The listing builds one solid part. Answer for the finished solid, in the listing's coordinates (mm). A direction names the side the tool comes from. Coordinates: 2 decimals unless noted, no trailing zeros. Write each loop counter-clockwise with the first axis right and the second up, starting at its lowest first coordinate (ties: lowest second). Pieces come first, ordered by that corner, then holes.
from build123d import *

# Parameters (mm, degrees)
SKETCH1_R           = 25.4
SKETCH1_R_2         = 3.175
BOSS_EXTRUDE1_DEPTH = 2.54
SKETCH2_R           = 3.175
BOSS_EXTRUDE4_DEPTH = 13.97
SKETCH5_R           = 3.175
BOSS_EXTRUDE6_DEPTH = 2.54
SKETCH5_4_R         = 11.1125
BOSS_EXTRUDE7_DEPTH = 8.89
SKETCH6_R           = 25.4
SKETCH6_R_2         = 11.1125
BOSS_EXTRUDE8_DEPTH = 2.54


with BuildPart() as part:
    # Sketch1 → Boss-Extrude1 (new body)
    with BuildSketch(Plane(origin=(0, 0, 0), x_dir=(1, 0, 0), z_dir=(0, 1, 0))):
        Circle(SKETCH1_R)
        Circle(SKETCH1_R_2, mode=Mode.SUBTRACT)
    extrude(amount=BOSS_EXTRUDE1_DEPTH)

    # Sketch2 → Boss-Extrude4 (add)
    with BuildSketch(Plane(origin=(0, 2.54, 0), x_dir=(1, 0, 0), z_dir=(0, 1, 0))):
        with BuildLine():
            ThreePointArc((0.635, 25.392061259), (0, 25.4), (-0.635, 25.392061259))
            Line((-0.635, 25.392061259), (-0.635, 4.719976827))
            ThreePointArc((-0.635, 4.719976827), (-1.822529847, 4.399976274), (-2.888514816, 3.786540428))
            Line((-2.888514816, 3.786540428), (-17.505885899, 18.403911511))
            ThreePointArc((-17.505885899, 18.403911511), (-17.960512242, 17.960512242), (-18.403911511, 17.505885899))
            Line((-18.403911511, 17.505885899), (-3.786540428, 2.888514816))
            ThreePointArc((-3.786540428, 2.888514816), (-4.399976274, 1.822529847), (-4.719976827, 0.635))
            Line((-4.719976827, 0.635), (-25.392061259, 0.635))
            ThreePointArc((-25.392061259, 0.635), (-25.4, 0), (-25.392061259, -0.635))
            Line((-25.392061259, -0.635), (-4.719976827, -0.635))
            ThreePointArc((-4.719976827, -0.635), (-4.399976274, -1.822529847), (-3.786540428, -2.888514816))
            Line((-3.786540428, -2.888514816), (-18.403911511, -17.505885899))
            ThreePointArc((-18.403911511, -17.505885899), (-17.960512242, -17.960512242), (-17.505885899, -18.403911511))
            Line((-17.505885899, -18.403911511), (-2.888514816, -3.786540428))
            ThreePointArc((-2.888514816, -3.786540428), (-1.822529847, -4.399976274), (-0.635, -4.719976827))
            Line((-0.635, -4.719976827), (-0.635, -25.392061259))
            ThreePointArc((-0.635, -25.392061259), (0, -25.4), (0.635, -25.392061259))
            Line((0.635, -25.392061259), (0.635, -4.719976827))
            ThreePointArc((0.635, -4.719976827), (1.822529847, -4.399976274), (2.888514816, -3.786540428))
            Line((2.888514816, -3.786540428), (17.505885899, -18.403911511))
            ThreePointArc((17.505885899, -18.403911511), (17.960512242, -17.960512242), (18.403911511, -17.505885899))
            Line((18.403911511, -17.505885899), (3.786540428, -2.888514816))
            ThreePointArc((3.786540428, -2.888514816), (4.399976274, -1.822529847), (4.719976827, -0.635))
            Line((4.719976827, -0.635), (25.392061259, -0.635))
            ThreePointArc((25.392061259, -0.635), (25.4, 0), (25.392061259, 0.635))
            Line((25.392061259, 0.635), (4.719976827, 0.635))
            ThreePointArc((4.719976827, 0.635), (4.399976274, 1.822529847), (3.786540428, 2.888514816))
            Line((3.786540428, 2.888514816), (18.403911511, 17.505885899))
            ThreePointArc((18.403911511, 17.505885899), (17.960512242, 17.960512242), (17.505885899, 18.403911511))
            Line((17.505885899, 18.403911511), (2.888514816, 3.786540428))
            ThreePointArc((2.888514816, 3.786540428), (1.822529847, 4.399976274), (0.635, 4.719976827))
            Line((0.635, 4.719976827), (0.635, 25.392061259))
        make_face()
        Circle(SKETCH2_R, mode=Mode.SUBTRACT)
    extrude(amount=BOSS_EXTRUDE4_DEPTH)

    # Sketch5 → Boss-Extrude6 (add)
    with BuildSketch(Plane(origin=(0, 16.51, 0), x_dir=(1, 0, 0), z_dir=(0, 1, 0))):
        with BuildLine():
            Line((3.786540428, -2.888514816), (8.293897485, -7.395871873))
            ThreePointArc((8.293897485, -7.395871873), (10.266611305, -4.252569642), (11.094342308, -0.635))
            Line((11.094342308, -0.635), (4.719976827, -0.635))
            ThreePointArc((4.719976827, -0.635), (4.399976274, -1.822529847), (3.786540428, -2.888514816))
        make_face()
        with BuildLine():
            ThreePointArc((-0.635, -11.094342308), (0, -11.1125), (0.635, -11.094342308))
            Line((0.635, -11.094342308), (0.635, -4.719976827))
            ThreePointArc((0.635, -4.719976827), (1.822529847, -4.399976274), (2.888514816, -3.786540428))
            Line((2.888514816, -3.786540428), (7.395871873, -8.293897485))
            ThreePointArc((7.395871873, -8.293897485), (7.857724106, -7.857724106), (8.293897485, -7.395871873))
            Line((8.293897485, -7.395871873), (3.786540428, -2.888514816))
            ThreePointArc((3.786540428, -2.888514816), (4.399976274, -1.822529847), (4.719976827, -0.635))
            Line((4.719976827, -0.635), (11.094342308, -0.635))
            ThreePointArc((11.094342308, -0.635), (11.107959649, -0.317629777), (11.1125, 0))
            ThreePointArc((11.1125, 0), (11.107959649, 0.317629777), (11.094342308, 0.635))
            Line((11.094342308, 0.635), (4.719976827, 0.635))
            ThreePointArc((4.719976827, 0.635), (4.399976274, 1.822529847), (3.786540428, 2.888514816))
            Line((3.786540428, 2.888514816), (8.293897485, 7.395871873))
            ThreePointArc((8.293897485, 7.395871873), (7.857724106, 7.857724106), (7.395871873, 8.293897485))
            Line((7.395871873, 8.293897485), (2.888514816, 3.786540428))
            ThreePointArc((2.888514816, 3.786540428), (1.822529847, 4.399976274), (0.635, 4.719976827))
            Line((0.635, 4.719976827), (0.635, 11.094342308))
            ThreePointArc((0.635, 11.094342308), (0, 11.1125), (-0.635, 11.094342308))
            Line((-0.635, 11.094342308), (-0.635, 4.719976827))
            ThreePointArc((-0.635, 4.719976827), (-1.822529847, 4.399976274), (-2.888514816, 3.786540428))
            Line((-2.888514816, 3.786540428), (-7.395871873, 8.293897485))
            ThreePointArc((-7.395871873, 8.293897485), (-7.857724106, 7.857724106), (-8.293897485, 7.395871873))
            Line((-8.293897485, 7.395871873), (-3.786540428, 2.888514816))
            ThreePointArc((-3.786540428, 2.888514816), (-4.399976274, 1.822529847), (-4.719976827, 0.635))
            Line((-4.719976827, 0.635), (-11.094342308, 0.635))
            ThreePointArc((-11.094342308, 0.635), (-11.1125, 0), (-11.094342308, -0.635))
            Line((-11.094342308, -0.635), (-4.719976827, -0.635))
            ThreePointArc((-4.719976827, -0.635), (-4.399976274, -1.822529847), (-3.786540428, -2.888514816))
            Line((-3.786540428, -2.888514816), (-8.293897485, -7.395871873))
            ThreePointArc((-8.293897485, -7.395871873), (-7.857724106, -7.857724106), (-7.395871873, -8.293897485))
            Line((-7.395871873, -8.293897485), (-2.888514816, -3.786540428))
            ThreePointArc((-2.888514816, -3.786540428), (-1.822529847, -4.399976274), (-0.635, -4.719976827))
            Line((-0.635, -4.719976827), (-0.635, -11.094342308))
        make_face()
        Circle(SKETCH5_R, mode=Mode.SUBTRACT)
        with BuildLine():
            Line((0.635, -4.719976827), (0.635, -11.094342308))
            ThreePointArc((0.635, -11.094342308), (4.252569642, -10.266611305), (7.395871873, -8.293897485))
            Line((7.395871873, -8.293897485), (2.888514816, -3.786540428))
            ThreePointArc((2.888514816, -3.786540428), (1.822529847, -4.399976274), (0.635, -4.719976827))
        make_face()
        with BuildLine():
            ThreePointArc((-7.395871873, -8.293897485), (-4.252569642, -10.266611305), (-0.635, -11.094342308))
            Line((-0.635, -11.094342308), (-0.635, -4.719976827))
            ThreePointArc((-0.635, -4.719976827), (-1.822529847, -4.399976274), (-2.888514816, -3.786540428))
            Line((-2.888514816, -3.786540428), (-7.395871873, -8.293897485))
        make_face()
        with BuildLine():
            ThreePointArc((-11.094342308, -0.635), (-10.266611305, -4.252569642), (-8.293897485, -7.395871873))
            Line((-8.293897485, -7.395871873), (-3.786540428, -2.888514816))
            ThreePointArc((-3.786540428, -2.888514816), (-4.399976274, -1.822529847), (-4.719976827, -0.635))
            Line((-4.719976827, -0.635), (-11.094342308, -0.635))
        make_face()
        with BuildLine():
            ThreePointArc((-8.293897485, 7.395871873), (-10.266611305, 4.252569642), (-11.094342308, 0.635))
            Line((-11.094342308, 0.635), (-4.719976827, 0.635))
            ThreePointArc((-4.719976827, 0.635), (-4.399976274, 1.822529847), (-3.786540428, 2.888514816))
            Line((-3.786540428, 2.888514816), (-8.293897485, 7.395871873))
        make_face()
        with BuildLine():
            ThreePointArc((-0.635, 11.094342308), (-4.252569642, 10.266611305), (-7.395871873, 8.293897485))
            Line((-7.395871873, 8.293897485), (-2.888514816, 3.786540428))
            ThreePointArc((-2.888514816, 3.786540428), (-1.822529847, 4.399976274), (-0.635, 4.719976827))
            Line((-0.635, 4.719976827), (-0.635, 11.094342308))
        make_face()
        with BuildLine():
            Line((2.888514816, 3.786540428), (7.395871873, 8.293897485))
            ThreePointArc((7.395871873, 8.293897485), (4.252569642, 10.266611305), (0.635, 11.094342308))
            Line((0.635, 11.094342308), (0.635, 4.719976827))
            ThreePointArc((0.635, 4.719976827), (1.822529847, 4.399976274), (2.888514816, 3.786540428))
        make_face()
        with BuildLine():
            Line((4.719976827, 0.635), (11.094342308, 0.635))
            ThreePointArc((11.094342308, 0.635), (10.266611305, 4.252569642), (8.293897485, 7.395871873))
            Line((8.293897485, 7.395871873), (3.786540428, 2.888514816))
            ThreePointArc((3.786540428, 2.888514816), (4.399976274, 1.822529847), (4.719976827, 0.635))
        make_face()
    extrude(amount=BOSS_EXTRUDE6_DEPTH)

    # Sketch5_4 → Boss-Extrude7 (add)
    with BuildSketch(Plane(origin=(0, 16.51, 0), x_dir=(1, 0, 0), z_dir=(0, 1, 0))):
        with BuildLine():
            Line((-0.635, -12.684115066), (-0.635, -25.392061259))
            ThreePointArc((-0.635, -25.392061259), (0, -25.4), (0.635, -25.392061259))
            Line((0.635, -25.392061259), (0.635, -12.684115066))
            ThreePointArc((0.635, -12.684115066), (4.860079591, -11.733270063), (8.52001097, -9.418036582))
            Line((8.52001097, -9.418036582), (17.505885899, -18.403911511))
            ThreePointArc((17.505885899, -18.403911511), (17.960512242, -17.960512242), (18.403911511, -17.505885899))
            Line((18.403911511, -17.505885899), (9.418036582, -8.52001097))
            ThreePointArc((9.418036582, -8.52001097), (11.733270063, -4.860079591), (12.684115066, -0.635))
            Line((12.684115066, -0.635), (25.392061259, -0.635))
            ThreePointArc((25.392061259, -0.635), (25.4, 0), (25.392061259, 0.635))
            Line((25.392061259, 0.635), (12.684115066, 0.635))
            ThreePointArc((12.684115066, 0.635), (11.733270063, 4.860079591), (9.418036582, 8.52001097))
            Line((9.418036582, 8.52001097), (18.403911511, 17.505885899))
            ThreePointArc((18.403911511, 17.505885899), (17.960512242, 17.960512242), (17.505885899, 18.403911511))
            Line((17.505885899, 18.403911511), (8.52001097, 9.418036582))
            ThreePointArc((8.52001097, 9.418036582), (4.860079591, 11.733270063), (0.635, 12.684115066))
            Line((0.635, 12.684115066), (0.635, 25.392061259))
            ThreePointArc((0.635, 25.392061259), (0, 25.4), (-0.635, 25.392061259))
            Line((-0.635, 25.392061259), (-0.635, 12.684115066))
            ThreePointArc((-0.635, 12.684115066), (-4.860079591, 11.733270063), (-8.52001097, 9.418036582))
            Line((-8.52001097, 9.418036582), (-17.505885899, 18.403911511))
            ThreePointArc((-17.505885899, 18.403911511), (-17.960512242, 17.960512242), (-18.403911511, 17.505885899))
            Line((-18.403911511, 17.505885899), (-9.418036582, 8.52001097))
            ThreePointArc((-9.418036582, 8.52001097), (-11.733270063, 4.860079591), (-12.684115066, 0.635))
            Line((-12.684115066, 0.635), (-25.392061259, 0.635))
            ThreePointArc((-25.392061259, 0.635), (-25.4, 0), (-25.392061259, -0.635))
            Line((-25.392061259, -0.635), (-12.684115066, -0.635))
            ThreePointArc((-12.684115066, -0.635), (-11.733270063, -4.860079591), (-9.418036582, -8.52001097))
            Line((-9.418036582, -8.52001097), (-18.403911511, -17.505885899))
            ThreePointArc((-18.403911511, -17.505885899), (-17.960512242, -17.960512242), (-17.505885899, -18.403911511))
            Line((-17.505885899, -18.403911511), (-8.52001097, -9.418036582))
            ThreePointArc((-8.52001097, -9.418036582), (-4.860079591, -11.733270063), (-0.635, -12.684115066))
        make_face()
        Circle(SKETCH5_4_R, mode=Mode.SUBTRACT)
    extrude(amount=BOSS_EXTRUDE7_DEPTH)

    # Sketch6 → Boss-Extrude8 (add)
    with BuildSketch(Plane(origin=(0, 25.4, 0), x_dir=(1, 0, 0), z_dir=(0, 1, 0))):
        Circle(SKETCH6_R)
        Circle(SKETCH6_R_2, mode=Mode.SUBTRACT)
    extrude(amount=BOSS_EXTRUDE8_DEPTH)


solid = part.part
Q1. Find the intervals of material crossed by probe 1 along X at (y, z) = (10, 0) (3 decimals); probe 2 along Y at (x, z) = (4.5, -19.5), in increasing order.
Answers below:
probe 1: x = -25.4 to -3.175, 3.175 to 25.4
probe 2: y = 0 to 2.54, 25.4 to 27.94
Q2. The part is cut by section D-D, the plane z = 12. Write down the section's boundary in (x, y) (3 decimals), then the cut area to 3 significant figures.
Answers below:
outline: (-22.387, 0) - (22.387, 0) - (22.387, 2.54) - (12.898, 2.54) - (12.898, 25.4) - (22.387, 25.4) - (22.387, 27.94) - (-22.387, 27.94) - (-22.387, 25.4) - (-12.898, 25.4) - (-12.898, 2.54) - (-22.387, 2.54) - close; hole (-11.102, 2.54) - (-0.635, 2.54) - (-0.635, 16.51) - (-4.158, 16.51) - (-4.158, 25.4) - (-11.102, 25.4) - close; hole (0.635, 2.54) - (11.102, 2.54) - (11.102, 25.4) - (4.158, 25.4) - (4.158, 16.51) - (0.635, 16.51) - close
area: 401 mm2
Q3. Determine the mould class of faces 4 (the face through (5, 0, 0)), 5 (the face through (-4.92, 20.89, 11.71)), 6 (the face through (11.76, 20.89, -4.8)) for opening direction Z: released by +Z, released by -Z, zero draft, split by the parting line, or undercut.
Answers below:
face 4: zero draft
face 5: released by +Z
face 6: undercut
Q4. Given pin 1 (6 mm diameter, centred on x = 5, z = 2, fed in from +Y); pin 2 (3 mm diameter, centred on y = 11, z = 11.5, fed in from +X); pin 3 (8 mm diameter, centred on y = 10.5, z = -20.5, fed in from -X); pin 4 (3 mm diameter, centred on x = 9, z = -0.5, fed in from -Y), each flat-ended and moving along its own axis, determine where each tip first touches the part or whether it passes through.
Answers below:
pin 1: stops at y = 19.05
pin 2: stops at x = 13.9
pin 3: stops at x = -18.4
pin 4: stops at y = 0
Q5. Which of the six approach directions +Z, -Z, +X, -X, +Y, -Y give full straight-line access (tool end or side, diameter ignored) to faces 1 (the face through (4.393, 9.427, 1.838)), 2 (the face through (-8, 16.51, -4)), 3 (the face through (-7, 25.4, 17))?
Answers below:
face 1: +X
face 2: -X
face 3: +Z
